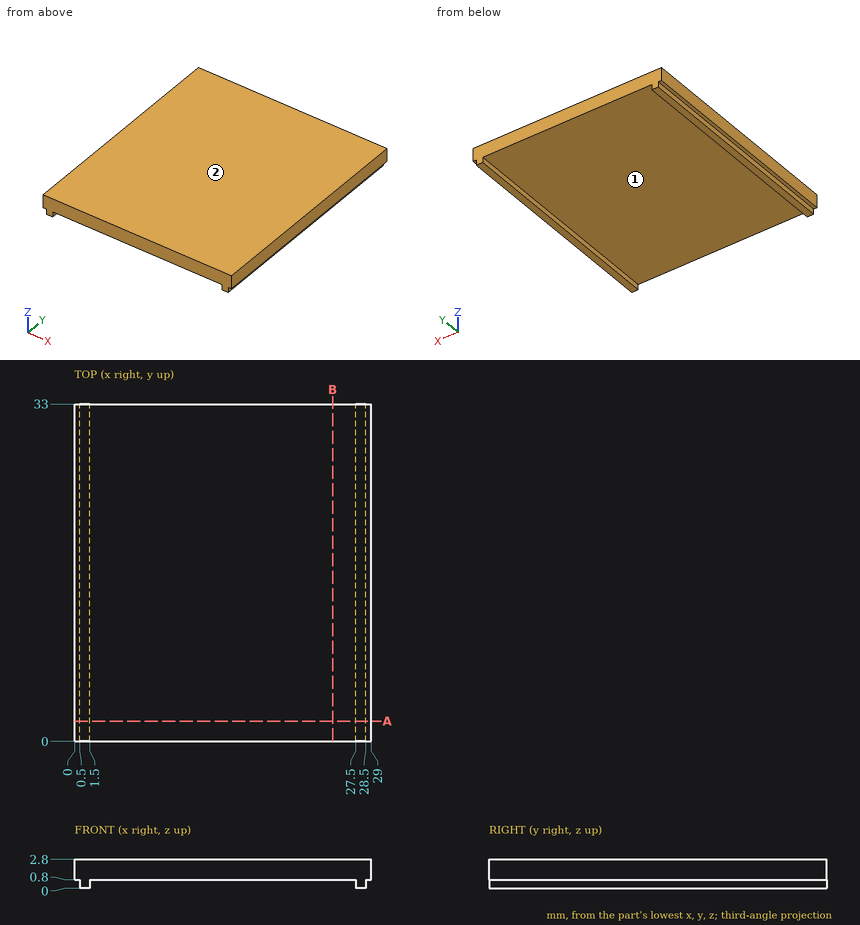
Print and shaded views of the part. All mm, measured from the part's lowest x, y and z. Coordinates: 2 decimals unless noted, no trailing zeros. Loops run counter-clockwise (first coordinate to the right, second up) from the corner with the lowest first, then second, coordinate; pieces in that order, holes last. Notation, with made-up numbers: (-32, 84) -> (-2, 84) arc R17 cw to (-2, 106) -> close; hole circle Ø11 at (-15, 68). An arc over 180 degrees is marked (long way). Use a Markdown table: item, result. Add a question column.
Item 1: Probe probe 1 along X at (y, z) = (11, 0.35); probe 2 along Z at (x, y) = (27.25, 26). List the from-to ranges inside material, lowest first.
Item 2: Pull direction X, two halves, no side cores. Call the marked faces 1 and 2: +X half, -X half, draft (parallel to the pull), parting line (faces both ways), or undercut.
Item 3: Band-saw the part on A-A on y = 2. Write the cut outline in (x, z), plus the area to 3 significant figures.
Item 4: Flat gauge pin, fed straight in: P1, Ø1, axis at x = 14.5, y = 23.5, coming from the -Z side. Where does the tip first touch, or does it go through?
Item 5: Band-saw the part on B-B on x = 25.25. Write the cut outline in (y, z), plus the area to 3 significant figures.
Geometry says:
| question | item | result |
|---|---|---|
| 1 | probe 1 | 0.5 to 1.5, 27.5 to 28.5 |
| 1 | probe 2 | 0.8 to 2.8 |
| 2 | face 1 | undercut |
| 2 | face 2 | draft |
| 3 | outline | (0, 0.8) -> (0.5, 0.8) -> (0.5, 0) -> (1.5, 0) -> (1.5, 0.8) -> (27.5, 0.8) -> (27.5, 0) -> (28.5, 0) -> (28.5, 0.8) -> (29, 0.8) -> (29, 2.8) -> (0, 2.8) -> close |
| 3 | area | 59.6 mm² |
| 4 | P1 | z = 0.8 |
| 5 | outline | (0, 0.8) -> (33, 0.8) -> (33, 2.8) -> (0, 2.8) -> close |
| 5 | area | 66.0 mm² |
